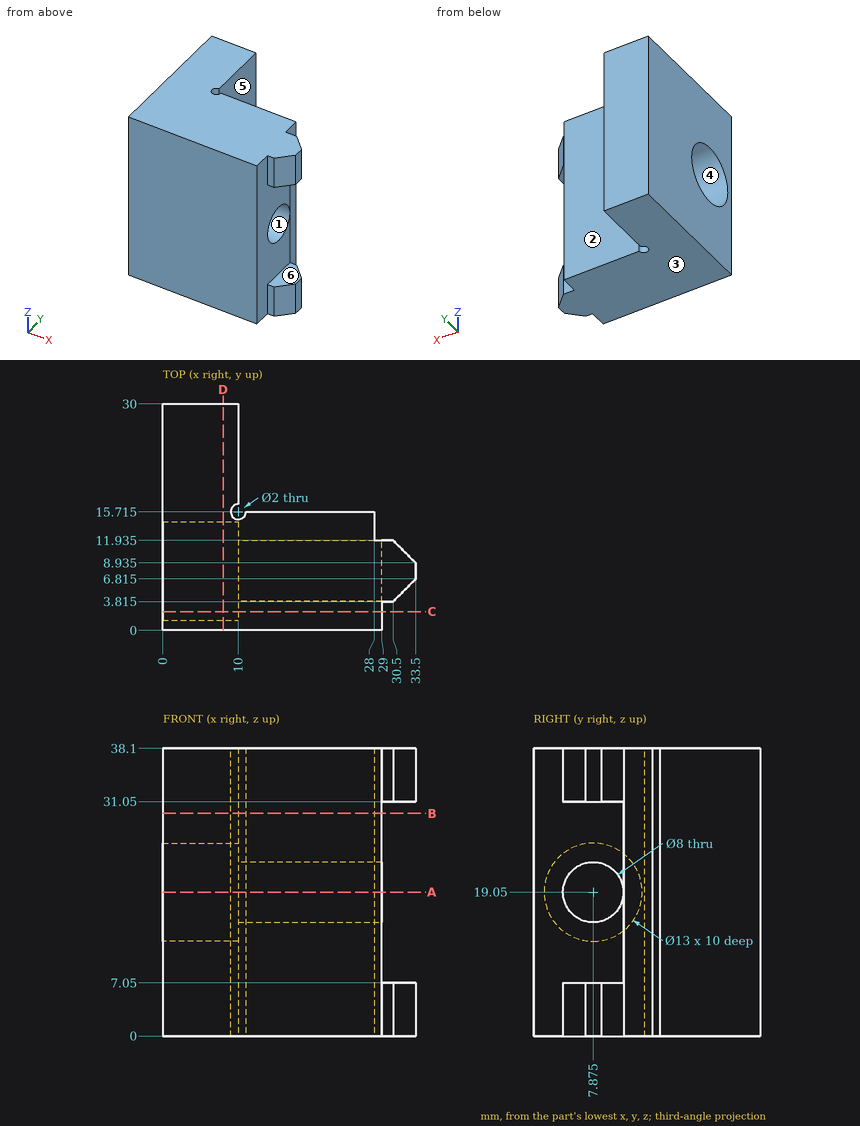
Input: dimensioned drawing with shaded views. Units: mm. Origin: part minimum x, y, z. A direction names the side the tool comes from. Coordinates: 2 decimals unless noted, no trailing zeros. Loops run counter-clockwise (first coordinate to the right, second up) from the corner with the lowest first, then second, coordinate; pieces in that order, holes last.
Q1. Line query: line 1 along Y through (x, z) = (14.75, 19.05) (3 decimals); line 2 along Z through (x, y) = (6, 7.5); line 3 along Y through (x, z) = (4, 19.05) (3 decimals). Output: solid intervals per line, ascending.
Results are:
line 1: y = 0 to 3.875, 11.875 to 15.715
line 2: z = 0 to 12.56, 25.54 to 38.1
line 3: y = 0 to 1.375, 14.375 to 30
Q2. Section A-A, the plane z = 19.05. Return the cut outline in (x, y) (3 decimals), and give its area (3 significant figures).
Results are:
outline: (0, 0) - (29, 0) - (29, 3.875) - (10, 3.875) - (10, 1.375) - (0, 1.375) - close; (0, 14.375) - (10, 14.375) - (10, 11.875) - (29, 11.875) - (29, 11.935) - (28, 11.935) - (28, 15.715) - (11, 15.715) arc R1 cw (long way) to (10, 16.715) - (10, 30) - (0, 30) - close
area: 310 mm2
Q3. Section B-B, the plane z = 29.5. Return the cut outline in (x, y) (3 decimals).
Results are:
outline: (0, 0) - (29, 0) - (29, 11.935) - (28, 11.935) - (28, 15.715) - (11, 15.715) arc R1 cw (long way) to (10, 16.715) - (10, 30) - (0, 30) - close
Q4. Section C-C, the plane y = 2.5. Return the cut outline in (x, z) (3 decimals).
Results are:
outline: (0, 0) - (29, 0) - (29, 38.1) - (0, 38.1) - (0, 22.705) - (10, 22.705) - (10, 15.395) - (0, 15.395) - close
Q5. Contact query for flat-ended pins moving along their axis: pin 1 (0.8 mm diameter, centred on x = 30, z = 2.5, fed in from -Y) (3 decimals); pin 2 (1.5 mm diameter, centred on x = 24.5, z = 6, fed in from +Y) (3 decimals); pin 3 (3 mm diameter, centred on y = 18, z = 21, fed in from +X); pin 4 (2 mm diameter, centred on x = 18, y = 15.5, fed in from -Z). Output: stop coordinate, or through.
Results are:
pin 1: stops at y = 3.815
pin 2: stops at y = 15.715
pin 3: stops at x = 10
pin 4: stops at z = 0
Q6. Set-up query: the marked faces 4, 5 and 6. Return all of +Z, -Z, +X, -X, +Y, -Y with unobstructed straight access to the full face (end or side cutting, diameter ignored); none if empty.
Results are:
face 4: -X
face 5: +Z, -Z, +X, +Y
face 6: +X, +Y, -Y
Q7. Section D-D, the plane x = 8. Return the cut outline in (y, z) (3 decimals), and give its area (3 significant figures).
Results are:
outline: (0, 0) - (30, 0) - (30, 38.1) - (0, 38.1) - close; hole circle Ø13 at (7.875, 19.05)
area: 1,010 mm2
Q8. Mould query, pull axis Y, two halves, no side actions, for the marked faces 1, 2 and 3. Classes: +Y half, -Y half, draft (parallel to the pull), parting line (faces both ways), or undercut.
Results are:
face 1: undercut
face 2: +Y half
face 3: draft
